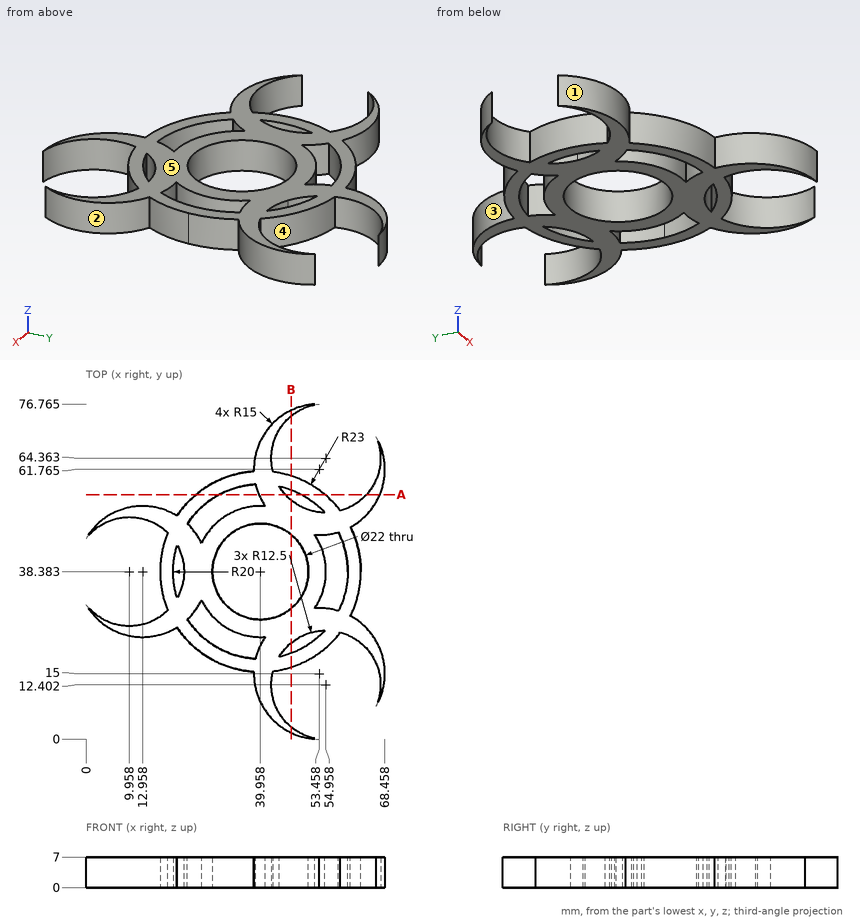
Geometry: see drawing. Coordinates: mm, zero at the bounding-box minimum. A direction names the side the tool comes from. Give positions to 0.01 mm unless a question says otherwise; leave off trailing zeros. Order: outer loops, then holes, each group sorted by start corner. A loop starts at its lowest first (then second) coordinate and runs counter-clockwise, first axis right, second up. Notation, with made-up numbers: (28.25, -25.75) - (68.25, -25.75) arc R16 ccw to (68.25, -12.75) - close; hole circle Ø1 at (-12.75, -8.75). An arc over 180 degrees is marked (long way). Write each question's results on one line, items separated by ' | '.
Item 1: Draft query along X for the marked faces 1, 2 and 3. Return one class per face: released by +X, released by -X, zero draft, split by the parting line, or undercut.
A:
face 1: undercut | face 2: released by +X | face 3: released by -X
Item 2: Section B-B (x = 47). Return loops of the section in (y, z), and give its area (3 significant figures).
A:
outline: (1.46, 0) - (2.76, 0) - (2.76, 7) - (1.46, 7) - close; (16.49, 0) - (19.66, 0) - (19.66, 7) - (16.49, 7) - close; (22.04, 0) - (29.93, 0) - (29.93, 7) - (22.04, 7) - close; (46.83, 0) - (54.72, 0) - (54.72, 7) - (46.83, 7) - close; (57.1, 0) - (60.28, 0) - (60.28, 7) - (57.1, 7) - close; (74, 0) - (75.3, 0) - (75.3, 7) - (74, 7) - close | area: 173 mm^2
Item 3: Contact query for flat-ended pins moving along their axis: pin 1 Ø4 at (x, z) = (60, 2) entering from +Y (1 decimal); pin 2 Ø1 at (x, z) = (33, 1.5) entering from -Y; pin 3 Ø1 at (x, z) = (31.5, 1) entering from +Y. Output: stop coordinate, or through.
A:
pin 1: stops at y = 54 | pin 2: stops at y = 16.31 | pin 3: stops at y = 59.96
Item 4: Access query for the marked faces 4 and 5. Directions: +Z, -Z, +X, -X, +Y, -Y. A direction counts if a zero-diameter tool reaches every point of the face in a straight line with its end or side. Return the directions, or none.
A:
face 4: +Z, -Z | face 5: +Z, +X, -X, +Y, -Y
Item 5: Material intervals for line 1 along X through (y, z) = (40.5, 5.5) (1 decimal); line 2 along X through (y, z) = (38.5, 3.25); line 3 along Y through (x, z) = (64, 1.5) (1 decimal), sorted ascending.
A:
line 1: x = 17.1 to 20.1, 22.3 to 29.2, 50.8 to 54.8, 59.8 to 62.9 | line 2: x = 16.96 to 19.96, 22.46 to 28.96, 50.96 to 54.96, 59.96 to 62.96 | line 3: y = 21 to 25.7, 51.1 to 55.7
Item 6: Section A-A (y = 56). Return loops of the section in (x, z) (1 decimal).
A:
outline: (25.2, 0) - (30.5, 0) - (30.5, 7) - (25.2, 7) - close; (39.6, 0) - (45.7, 0) - (45.7, 7) - (39.6, 7) - close; (49.4, 0) - (54.7, 0) - (54.7, 7) - (49.4, 7) - close; (64.2, 0) - (67.3, 0) - (67.3, 7) - (64.2, 7) - close
